from build123d import *

# Parameters (mm, degrees)
SKETCH_W        = 85
SKETCH_H        = 56
PAD_DEPTH       = 2
SKETCH001_R     = 3
PAD001_DEPTH    = 5
FILLET_R        = 3
SKETCH002_R     = 0.5
POCKET_DEPTH    = 5
SKETCH003_R     = 0.5
POCKET001_DEPTH = 5
SKETCH004_R     = 0.5
POCKET002_DEPTH = 5
SKETCH005_R     = 0.5
POCKET003_DEPTH = 5
POCKET004_DEPTH = 2.001


with BuildPart() as part:
    # Sketch → Pad (new body)
    with BuildSketch(Plane.XY):
        with Locations((42.5, 28)):
            Rectangle(SKETCH_W, SKETCH_H)
    extrude(amount=PAD_DEPTH)

    # Sketch001 (on Face6 of Pad) → Pad001 (join)
    with BuildSketch(Plane.XY.offset(2)):
        with Locations((3.5, 3.5)):
            Circle(SKETCH001_R)
        with Locations((3.5, 52.5)):
            Circle(SKETCH001_R)
        with Locations((61.5, 52.5)):
            Circle(SKETCH001_R)
        with Locations((61.5, 3.5)):
            Circle(SKETCH001_R)
    extrude(amount=PAD001_DEPTH)

    # Fillet
    fillet_edges = [part.edges().sort_by_distance(p)[0] for p in [
        (85, 0, 1),
        (85, 56, 1),
        (0, 56, 1),
        (0, 0, 1),
    ]]
    fillet(fillet_edges, radius=FILLET_R)

    # Sketch002 (on Face16 of Fillet) → Pocket (cut)
    with BuildSketch(Plane.XY.offset(7)):
        with Locations((3.5, 3.5)):
            Circle(SKETCH002_R)
    extrude(amount=-POCKET_DEPTH, mode=Mode.SUBTRACT)

    # Sketch003 (on Face17 of Pocket) → Pocket001 (cut)
    with BuildSketch(Plane.XY.offset(7)):
        with Locations((3.5, 52.5)):
            Circle(SKETCH003_R)
    extrude(amount=-POCKET001_DEPTH, mode=Mode.SUBTRACT)

    # Sketch004 (on Face15 of Pocket001) → Pocket002 (cut)
    with BuildSketch(Plane.XY.offset(7)):
        with Locations((61.5, 3.5)):
            Circle(SKETCH004_R)
    extrude(amount=-POCKET002_DEPTH, mode=Mode.SUBTRACT)

    # Sketch005 (on Face18 of Pocket002) → Pocket003 (cut)
    with BuildSketch(Plane.XY.offset(7)):
        with Locations((61.5, 52.5)):
            Circle(SKETCH005_R)
    extrude(amount=-POCKET003_DEPTH, mode=Mode.SUBTRACT)

    # Sketch006 (on Face5 of Pocket003) → Pocket004 (cut, through all)
    with BuildSketch(Plane.XY.offset(2)):
        with BuildLine():
            Line((10.571068, 49.5), (54.428932, 49.5))
            ThreePointArc((58.5, 45.428932), (57.307612, 48.307612), (54.428932, 49.5))
            Line((58.5, 45.428932), (58.5, 10.571068))
            ThreePointArc((54.428932, 6.5), (57.307612, 7.692388), (58.5, 10.571068))
            Line((54.428932, 6.5), (10.571068, 6.5))
            ThreePointArc((6.5, 10.571068), (7.692388, 7.692388), (10.571068, 6.5))
            Line((6.5, 10.571068), (6.5, 45.428932))
            ThreePointArc((10.571068, 49.5), (7.692388, 48.307612), (6.5, 45.428932))
        make_face()
        with BuildLine():
            Line((68.571068, 49.5), (74.191068, 49.5))
            ThreePointArc((78.5, 45.191068), (77.237943, 48.237943), (74.191068, 49.5))
            Line((78.5, 45.191068), (78.5, 10.571068))
            ThreePointArc((74.428932, 6.5), (77.307612, 7.692388), (78.5, 10.571068))
            Line((74.428932, 6.5), (68.571068, 6.5))
            ThreePointArc((64.5, 10.571068), (65.692388, 7.692388), (68.571068, 6.5))
            Line((64.5, 10.571068), (64.5, 45.428932))
            ThreePointArc((68.571068, 49.5), (65.692388, 48.307612), (64.5, 45.428932))
        make_face()
    extrude(amount=-POCKET004_DEPTH, mode=Mode.SUBTRACT)


solid = part.part
Input: part model. Units: mm. Frame: model coordinates. A direction names the side the tool comes from. Give positions to 0.01 mm unless a question says otherwise; leave off trailing zeros. Write each loop counter-clockwise with the first axis right and the second up, starting at its lowest first coordinate (ties: lowest second). Pieces come first, ordered by that corner, then holes.
Q1. Pull-direction query (X, two-part tool) for faces 4 (the face through (42, 56, 1)), 5 (the face through (0.86, 55.1, 1.01)), 6 (the face through (58.5, 28, 1)); classes: pulls with the +X half, pulls with the -X half, needs draft (parallel to the pull), parting line crosses it, or undercut.
Q2. Material intervals for probe 1 along Y at (x, z) = (3.5, 3.6); probe 2 along X at (y, z) = (33, 1.5); probe 3 along Y at (x, z) = (20, 1.75), sorted ascending.
Q3. First-contact query: P1, Ø1.5, axis at y = 6, z = 4.5, coming from the -X side; P2, Ø0.5, axis at x = 3.5, y = 3.5, coming from the +Z side. Flat tips, straight axial feed; report the tip coordinate or a pass-through.
Q4. Section A-A, the plane z = 4. Output: boundary loops of the cut face in (x, y).
Q5. Set-up query: faces 1 (the face through (4, 4, 7)), 2 (the face through (59.29, 54.53, 4.46)), 3 (the face through (6.5, 28, 1)). Return all of +Z, -Z, +X, -X, +Y, -Y with unobstructed straight access to the full face (end or side cutting, diameter ignored); none if empty.
Q6. Section B-B, the plane x = 12. Output: boundary loops of the cut face in (y, z).
Q7. Section C-C, the plane y = 36. Output: boundary loops of the cut face in (x, z).
Filled in:
1. face 4: needs draft
1. face 5: pulls with the -X half
1. face 6: undercut
2. probe 1: y = 0.5 to 3, 4 to 6.5, 49.5 to 52, 53 to 55.5
2. probe 2: x = 0 to 6.5, 58.5 to 64.5, 78.5 to 85
2. probe 3: y = 0 to 6.5, 49.5 to 56
3. P1: stops at x = 1.06
3. P2: stops at z = 2
4. outline: circle Ø6 at (3.5, 3.5); circle Ø6 at (3.5, 52.5); circle Ø6 at (61.5, 3.5); circle Ø6 at (61.5, 52.5); hole circle Ø1 at (3.5, 3.5); hole circle Ø1 at (3.5, 52.5); hole circle Ø1 at (61.5, 3.5); hole circle Ø1 at (61.5, 52.5)
5. face 1: +Z, +X, -X, +Y, -Y
5. face 2: +Z
5. face 3: +Z, -Z
6. outline: (0, 0) - (6.5, 0) - (6.5, 2) - (0, 2) - close; (49.5, 0) - (56, 0) - (56, 2) - (49.5, 2) - close
7. outline: (0, 0) - (6.5, 0) - (6.5, 2) - (0, 2) - close; (58.5, 0) - (64.5, 0) - (64.5, 2) - (58.5, 2) - close; (78.5, 0) - (85, 0) - (85, 2) - (78.5, 2) - close
